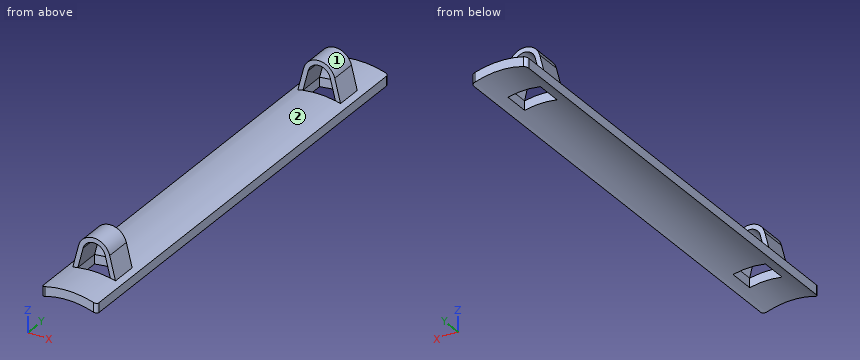
from build123d import *

# Parameters (mm, degrees)
PROFILE_DEPTH    = 35
SUPPORTCUTS_W    = 5
SUPPORTCUTS_H    = 4
SUPPORTCUT_DEPTH = 38.898185972
RODGUIDE_DEPTH   = 4
PROFILEFILLET_R  = 0.5


with BuildPart() as part:
    # ProfileS → Profile (new, symmetric)
    with BuildSketch(Plane(origin=(0, 0, 0), x_dir=(1, 0, 0), z_dir=(0, 1, 0))):
        with BuildLine():
            Line((-4.25, -11.755317946), (-4.25, -13.234330357))
            ThreePointArc((-4.25, -13.234330357), (0, -13.9), (4.25, -13.234330357))
            Line((4.25, -13.234330357), (4.25, -11.755317946))
            ThreePointArc((4.25, -11.755317946), (0, -12.5), (-4.25, -11.755317946))
        make_face()
    extrude(amount=PROFILE_DEPTH, both=True)

    # SupportCutS → SupportCut (cut, through all)
    with BuildSketch(Plane.XY):
        with Locations((0, 27)):
            Rectangle(SUPPORTCUTS_W, SUPPORTCUTS_H)
    supportcut = extrude(amount=SUPPORTCUT_DEPTH, mode=Mode.SUBTRACT)

    # RodGuideS → RodGuide (add)
    with BuildSketch(Plane.XZ.offset(-29)):
        with BuildLine():
            Line((-2.5, 13.673331708), (-1.696790343, 16.855729335))
            ThreePointArc((-1.696790343, 16.855729335), (0, 18.177474117), (1.696790343, 16.855729335))
            Line((1.696790343, 16.855729335), (2.5, 13.673331708))
            ThreePointArc((2.5, 13.673331708), (2.894968306, 13.5951888), (3.287507688, 13.505639311))
            Line((3.287507688, 13.505639311), (2.397347452, 17.032543895))
            ThreePointArc((2.397347452, 17.032543895), (0, 18.9), (-2.397347452, 17.032543895))
            Line((-2.397347452, 17.032543895), (-3.287507688, 13.505639311))
            ThreePointArc((-3.287507688, 13.505639311), (-2.894968306, 13.5951888), (-2.5, 13.673331708))
        make_face()
    rodguide = extrude(amount=RODGUIDE_DEPTH)

    # SCVM: SupportCut, RodGuide across plane
    add(supportcut.mirror(Plane.ZX), mode=Mode.SUBTRACT)
    add(rodguide.mirror(Plane.ZX))

    # ProfileFillet
    profilefillet_edges = [part.edges().sort_by_distance(p)[0] for p in [
        (4.25, 35, 12.494824151),
        (4.25, -35, 12.494824151),
        (-4.25, -35, 12.494824151),
        (-4.25, 35, 12.494824151),
    ]]
    fillet(profilefillet_edges, radius=PROFILEFILLET_R)


solid = part.part
Build history of the part. All positions in model axes, mm. Face numbers are marked on the shaded views. A direction names the side the tool comes from. Give positions to 0.01 mm unless a question says otherwise; leave off trailing zeros. Write each loop counter-clockwise with the first axis right and the second up, starting at its lowest first coordinate (ties: lowest second). Pieces come first, ordered by that corner, then holes. Notation, with made-up numbers: (55.5, 58) - (71.5, 58) arc R30 ccw to (71.5, 92) - close; hole circle Ø11 at (-31.75, -36). An arc over 180 degrees is marked (long way). Use one line per item in the form item = value. Start each with the question number.
1. Band-saw the part on B-B on y = -28. Write the cut outline in (x, z), plus the area to 3 significant figures.
2. Probe line 1 (Y direction, x = 0.25, z = 13.75); line 2 (Y direction, x = -1.25, z = 18); line 3 (Z direction, x = -0.25, y = 3.5). List the from-to ranges inside material, lowest first. Write a range as [from, to].
3. Band-saw the part on C-C on x = 1. Write the cut outline in (y, z).
4. Drop flat-ended pins along their axis: pin 1 Ø1.6 at (x, z) = (-0.5, 15.5) entering from +Y; pin 2 Ø2.5 at (x, z) = (-1.5, 16.5) entering from +Y; pin 3 Ø2.5 at (x, z) = (1, 17) entering from -Y. Give the stop position or say it passes through.
5. Band-saw the part on A-A on z = 14.75. Write the cut outline in (x, y), plus the area to 3 significant figures.
6. 3-axis set-ups, long thin cutter, end or side, ignore diameter. For the marked faces 1 and 2: which of +Z, -Z, +X, -X, +Y, -Y reach the whole face in a straight line?
Conclusion:
q1.outline = (-4.25, 11.76) arc R12.5 cw to (-2.5, 12.25) - (-2.5, 13.67) - (-1.7, 16.86) arc R1.75 cw to (1.7, 16.86) - (2.5, 13.67) - (2.5, 12.25) arc R12.5 cw to (4.25, 11.76) - (4.25, 13.23) arc R13.9 ccw to (3.29, 13.51) - (2.4, 17.03) arc R2.47 ccw to (-2.4, 17.03) - (-3.29, 13.51) arc R13.9 ccw to (-4.25, 13.23) - close
q1.area = 14.1 mm²
q2.line_1 = [-35, -29], [-25, 25], [29, 35]
q2.line_2 = [-29, -25], [25, 29]
q2.line_3 = [12.5, 13.9]
q3.outline = (-35, 12.46) - (-29, 12.46) - (-29, 13.86) - (-35, 13.86) - close; (-29, 17.86) - (-25, 17.86) - (-25, 18.69) - (-29, 18.69) - close; (-25, 12.46) - (25, 12.46) - (25, 13.86) - (-25, 13.86) - close; (25, 17.86) - (29, 17.86) - (29, 18.69) - (25, 18.69) - close; (29, 12.46) - (35, 12.46) - (35, 13.86) - (29, 13.86) - close
q4.pin_1 = through
q4.pin_2 = 29
q4.pin_3 = -29
q5.outline = (-2.97, -29) - (-2.23, -29) - (-2.23, -25) - (-2.97, -25) - close; (-2.97, 25) - (-2.23, 25) - (-2.23, 29) - (-2.97, 29) - close; (2.23, -29) - (2.97, -29) - (2.97, -25) - (2.23, -25) - close; (2.23, 25) - (2.97, 25) - (2.97, 29) - (2.23, 29) - close
q5.area = 11.9 mm²
q6.face_1 = +Z, +Y, -Y
q6.face_2 = +Z
